from build123d import *

# Parameters (mm, degrees)
SKETCH2_R           = 175
BOSS_EXTRUDE1_DEPTH = 15
SKETCH3_R           = 4
SKETCH3_R_2         = 50
CUT_EXTRUDE1_DEPTH  = 30


with BuildPart() as part:
    # Sketch2 → Boss-Extrude1 (new, symmetric)
    with BuildSketch(Plane(origin=(0, 0, 0), x_dir=(1, 0, 0), z_dir=(0, 1, 0))):
        with Locations(Location((0, 0, 0), (0, 0, 270))):
            Circle(SKETCH2_R)
    extrude(amount=BOSS_EXTRUDE1_DEPTH, both=True)

    # Sketch3 → Cut-Extrude1 (cut)
    with BuildSketch(Plane(origin=(0, 15, 0), x_dir=(1, 0, 0), z_dir=(0, 1, 0))):
        with Locations(Location((0, 160, 0), (0, 0, 270))):
            Circle(SKETCH3_R)
        with Locations(Location((0, -160, 0), (0, 0, 90))):
            Circle(SKETCH3_R)
        with Locations(Location((-160, 0, 0), (0, 0, 270))):
            Circle(SKETCH3_R)
        with Locations(Location((160, 0, 0), (0, 0, 90))):
            Circle(SKETCH3_R)
        with Locations(Location((0, 0, 0), (0, 0, 270))):
            Circle(SKETCH3_R_2)
    extrude(amount=-CUT_EXTRUDE1_DEPTH, mode=Mode.SUBTRACT)


solid = part.part
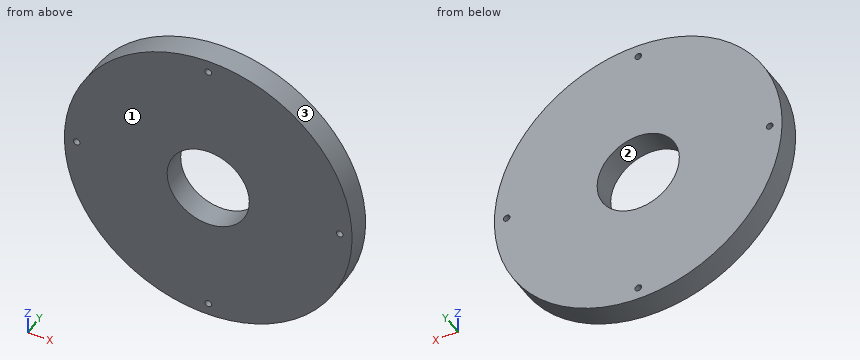
Geometry check sheet. Reference: the model listing, model coordinates, mm. Face numbers are marked on the shaded views. Coordinates: 2 decimals unless noted, no trailing zeros. Order: outer loops, then holes, each group sorted by start corner. A loop starts at its lowest first (then second) coordinate and runs counter-clockwise, first axis right, second up. Notation, with made-up numbers: (30.5, 60) -> (42.5, 60) arc R20 ccw to (42.5, 73) -> close; hole circle Ø5 at (78.25, 24.5). An arc over 180 degrees is marked (long way). Use a Markdown table: item, result. Add a question column.
1. Cross-section at C-C (x = 0). Enter the section's corners in (y, z), and give its area (3 significant figures).
2. Cross-section at D-D (z = 160). Enter the section's corners in (x, y).
3. Go/stop test with flat-tipped pins: pin 1 Ø10 at (x, y) = (129, 11) entering from +Z; pin 2 Ø2 at (y, z) = (8.5, -36.5) entering from +X; pin 3 Ø1 at (y, z) = (5.5, 70) entering from +X. Record where each tip stops, or that it passes through.
4. Cross-section at A-A (z = 0). Enter the section's corners in (x, y), and give its area (3 significant figures).
5. Cross-section at B-B (y = -10.75). Enter the section's corners in (x, z).
6. Mould release check, pull along X, two halves, no side actions. Record for the marked faces 1, 2 and 3: pulls with the +X half, pulls with the -X half, needs draft (parallel to the pull), parting line crosses it, or undercut.
7. Material ranges on L1, parallel to X at y = 6, z = 0; L2, parallel to Z at x = 160, y = 4.25, recorded low to high.
Filled sheet:
| question | item | result |
|---|---|---|
| 1 | outline | (-15, -175) -> (15, -175) -> (15, -164) -> (-15, -164) -> close; (-15, -156) -> (15, -156) -> (15, -50) -> (-15, -50) -> close; (-15, 50) -> (15, 50) -> (15, 156) -> (-15, 156) -> close; (-15, 164) -> (15, 164) -> (15, 175) -> (-15, 175) -> close |
| 1 | area | 7,020 mm2 |
| 2 | outline | (-70.89, -15) -> (-4, -15) -> (-4, 15) -> (-70.89, 15) -> close; (4, -15) -> (70.89, -15) -> (70.89, 15) -> (4, 15) -> close |
| 3 | pin 1 | z = 123.49 |
| 3 | pin 2 | x = 171.36 |
| 3 | pin 3 | x = 160.61 |
| 4 | outline | (-175, -15) -> (-164, -15) -> (-164, 15) -> (-175, 15) -> close; (-156, -15) -> (-50, -15) -> (-50, 15) -> (-156, 15) -> close; (50, -15) -> (156, -15) -> (156, 15) -> (50, 15) -> close; (164, -15) -> (175, -15) -> (175, 15) -> (164, 15) -> close |
| 4 | area | 7,020 mm2 |
| 5 | outline | circle Ø350 at (0, 0); hole circle Ø8 at (-160, 0); hole circle Ø100 at (0, 0); hole circle Ø8 at (0, -160); hole circle Ø8 at (0, 160); hole circle Ø8 at (160, 0) |
| 6 | face 1 | needs draft |
| 6 | face 2 | undercut |
| 6 | face 3 | parting line crosses it |
| 7 | L1 | -175 to -164, -156 to -50, 50 to 156, 164 to 175 |
| 7 | L2 | -70.89 to -4, 4 to 70.89 |
